```python
from build123d import *

# Parameters (mm, degrees)
F1_DEPTH       = 40
F3_D           = 3
F3_DEPTH       = 40
F3_CSINK_D     = 6
F3_CSINK_ANGLE = 90
F3_TIP         = 0.9012909285
F4_START       = -2.5
F2_W           = 98.723
F2_H           = 3.5
F4_DEPTH       = 98.5
F5_R           = 2


with BuildPart() as f1:
    # F0 (on Front) → F1 (new body)
    with BuildSketch(Plane.XZ):
        Polygon((53.7955448006, 85.2875881677), (53.7992331499, 4.6113628414), (-65.2007668501, 4.6113628414), (-65.2007668501, -1.3886371586), (60.0222331499, -1.3886371586), (60.0183739277, 83.0251359205), (111.0902979443, 134.055520892), (106.8493191704, 138.2998228416), align=None)
    extrude(amount=F1_DEPTH)

    # F3
    with Locations(Plane(origin=(0, 0, -1.3886371586), x_dir=(1, 0, 0), z_dir=(0, 0, -1))):
        with Locations((-50.2007668501, 33.75), (-50.2007668501, 6.25), (-18.2007668501, 6.25), (-18.2007668501, 33.75)):
            CounterSinkHole(F3_D / 2, F3_CSINK_D / 2, depth=F3_DEPTH, counter_sink_angle=F3_CSINK_ANGLE)
            with Locations((0, 0, -(F3_DEPTH + F3_TIP / 2))):  # 118° drill point
                Cone(0, F3_D / 2, F3_TIP, mode=Mode.SUBTRACT)

    # F2 (on face) → F4 (cut)
    with BuildSketch(Plane(origin=(0, 0, -1.3886371586), x_dir=(1, 0, 0), z_dir=(0, 0, -1)).offset(F4_START)):
        with Locations((7.1607331499, 20)):
            Rectangle(F2_W, F2_H)
    extrude(amount=-F4_DEPTH, mode=Mode.SUBTRACT)

    # F5
    f5_edges = [f1.edges().sort_by_distance(p)[0] for p in [
        (53.797389, -21.75, 44.949476),
        (53.799233, -30.875, 4.611363),
        (53.797389, -40, 44.949476),
        (53.795545, -30.875, 85.287588),
        (53.797389, 0, 44.949476),
        (53.799233, -9.125, 4.611363),
        (53.797389, -18.25, 44.949476),
        (53.795545, -9.125, 85.287588),
        (-65.200767, -20, 4.611363),
        (-65.200767, -20, -1.388637),
        (-65.200767, 0, 1.611363),
        (-65.200767, -40, 1.611363),
        (-5.700767, 0, 4.611363),
        (-2.589267, 0, -1.388637),
        (60.020304, 0, 40.818249),
        (85.554336, 0, 108.540328),
        (108.969809, 0, 136.177672),
        (80.322432, 0, 111.793706),
        (-5.700767, -40, 4.611363),
        (-2.589267, -40, -1.388637),
        (60.020304, -40, 40.818249),
        (85.554336, -40, 108.540328),
        (108.969809, -40, 136.177672),
        (80.322432, -40, 111.793706),
        (55.158889, -18.25, 86.649865),
        (56.522233, -20, 88.012142),
        (55.158889, -21.75, 86.649865),
        (106.849319, -20, 138.299823),
        (111.090298, -20, 134.055521),
        (60.022233, -20, -1.388637),
        (60.018374, -20, 83.025136),
        (5.799233, -21.75, 4.611363),
        (5.799233, -18.25, 4.611363),
    ]]
    fillet(f5_edges, radius=F5_R)


solid = f1.part
```
The model under review builds one solid part; all positions refer to its coordinate system, in mm. A direction names the side the tool comes from. Give positions to 0.01 mm unless a question says otherwise; leave off trailing zeros. Write each loop counter-clockwise with the first axis right and the second up, starting at its lowest first coordinate (ties: lowest second). Pieces come first, ordered by that corner, then holes. Notation, with made-up numbers: M 70.5,14 L 89.5,14 A31 cw 89.5,45 Z; hole C -24.5,31 d3. An arc over 180 degrees is marked long. Answer in a Markdown table with one row per item.
Item 1: For P1, Ø6, axis at x = -36, y = -36, coming from the +Z side; P2, Ø10, axis at y = -11, z = 21, coming from the +X side; P3, Ø10, axis at x = 74.5, y = -26.5, coming from the -Z side, all flat-tipped, find the tip position at first contact; note any pin that passes through.
Check sheet entries:
| item | result |
|---|---|
| P1 | z = 4.61 |
| P2 | x = 60.02 |
| P3 | z = 92.5 |
Item 2: Add section A-A on x = 43.5. Give the boundary of the cut face in (y, z), plus the area to 3 significant figures.
Check sheet entries:
| item | result |
|---|---|
| outline | M -40,0.61 A2 ccw -38,-1.39 L -2,-1.39 A2 ccw 0,0.61 L 0,2.61 A2 ccw -2,4.61 L -16.25,4.61 A2 ccw -18.25,2.61 L -18.25,1.11 L -21.75,1.11 L -21.75,2.61 A2 ccw -23.75,4.61 L -38,4.61 A2 ccw -40,2.61 Z |
| area | 223 mm2 |
Item 3: Tool access review of faces 4 (the face through (-42.201, -20, 3)), 5 (the face through (79.98, -0.57, 110.6)): name each direction out of +Z, -Z, +X, -X, +Y, -Y from which nothing blocks a thin tool from reaching the whole face with its end or side.
Check sheet entries:
| item | result |
|---|---|
| face 4 | +Z |
| face 5 | +Z, -X, +Y |
Item 4: Draft analysis for pull direction Y (two halves, no side actions). For faces 1 (the face through (6, -20, 1.111)), 2 (the face through (80.27, -19.75, 111.74)), 3 (the face through (85.081, -39.399, 108.873)), state which applies: +Y half, -Y half, draft (parallel to the pull), parting line (faces both ways), or undercut.
Check sheet entries:
| item | result |
|---|---|
| face 1 | undercut |
| face 2 | draft |
| face 3 | -Y half |
Item 5: For line 1 along X through (y, z) = (-33.75, 2.75); line 2 along X through (y, z) = (-6.5, 27); line 3 along Z through (x, y) = (-12.5, -28), list the stretches that pass through material, from the lowest coordinate up.
Check sheet entries:
| item | result |
|---|---|
| line 1 | -65.2 to -51.7, -48.7 to -19.7, -16.7 to 60.02 |
| line 2 | 53.8 to 60.02 |
| line 3 | -1.39 to 4.61 |
